Here's the drawing with two shaded views (mm, measured from the low corner). I have some questions. A direction names the side the tool comes from. Give positions to 0.01 mm unless a question says otherwise; leave off trailing zeros. Loops run counter-clockwise (first coordinate to the right, second up) from the corner with the lowest first, then second, coordinate; pieces in that order, holes last. Notation, with made-up numbers: (-39, 87) - (-32, 87) arc R23 cw to (-32, 111) - close; hole circle Ø9 at (2.25, 1). An arc over 180 degrees is marked (long way). Write each question's results on one line, items separated by ' | '. Start each with the question number.
1) If I drill on probe 1 along Y at (x, z) = (3, 1.9); probe 2 along Z at (x, y) = (3.1, 5.75); probe 3 along X at (y, z) = (3.35, 1.2), over which ranges is the centre line in solid material (lowest first)? Write a range as [from, to].
2) I'm going to push flat-ended pins straight in: pin 1 (3 mm diameter, centred on x = 3.5, y = 5, fed in from -Z); pin 2 (1 mm diameter, centred on y = 1, z = 2, fed in from +X); pin 3 (2 mm diameter, centred on y = 2, z = 4.5, fed in from +X). Where does each tip first touch, or does it pass through?
3) I want a section at A-A, the plane x = 3. Write out the boundary of the cut face in (y, z).
4) If we mould it in two halves opening along Y, with no side actions, what happens to the marked faces 1, 2 and 3? For each: +Y half, -Y half, draft (parallel to the pull), parting line (faces both ways), or undercut.
5) I want a section at C-C, the plane z = 4.35. Write out the boundary of the cut face in (x, y), and give its area (3 significant figures).
6) On a 3-axis mill with a long thin cutter (end or side, diameter ignored), from which of +Z, -Z, +X, -X, +Y, -Y can I reach the whole of each face in a straight line? I mean the marked faces 4 and 5. Say none if no direction works.
7) I want a section at D-D, the plane z = 1.2. Write out the boundary of the cut face in (x, y), and give its area (3 significant figures).
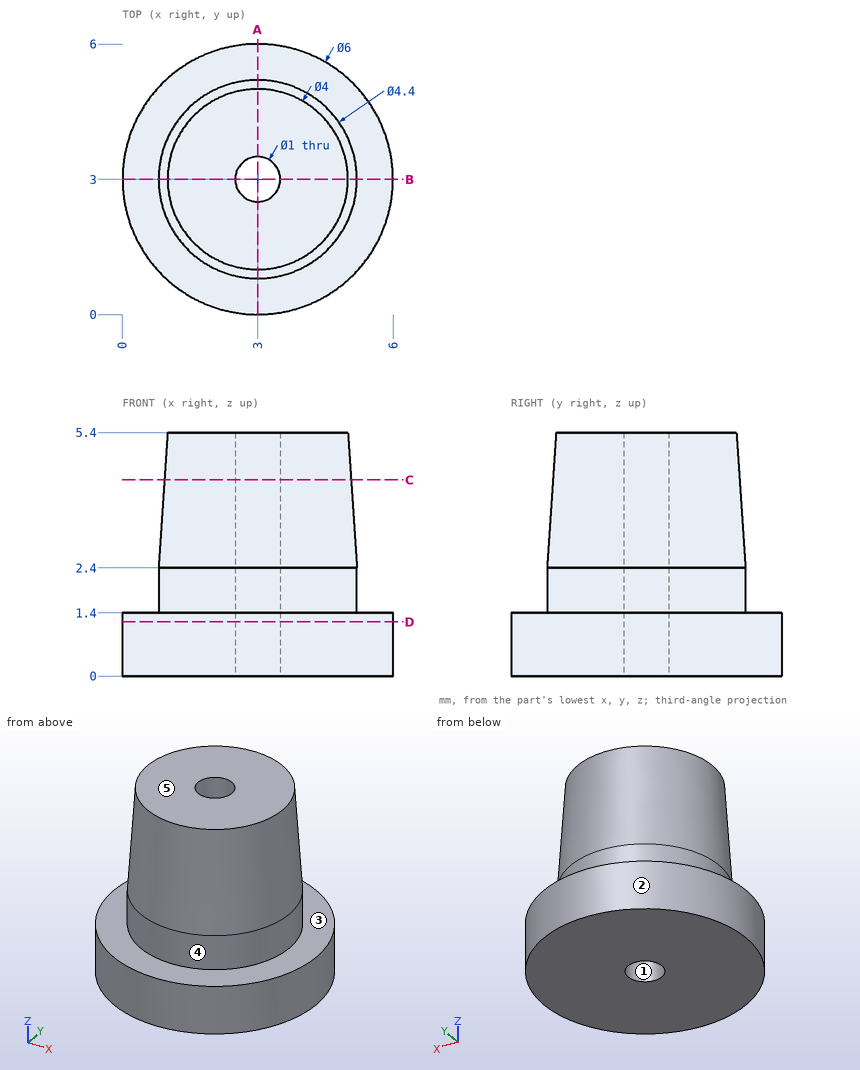
Answers:
1) probe 1: y = [0.8, 2.5], [3.5, 5.2] | probe 2: z = [0, 1.4] | probe 3: x = [0.02, 2.64], [3.36, 5.98]
2) pin 1: stops at z = 0 | pin 2: stops at x = 4.61 | pin 3: stops at x = 5.09
3) outline: (0, 0) - (2.5, 0) - (2.5, 5.4) - (1, 5.4) - (0.8, 2.4) - (0.8, 1.4) - (0, 1.4) - close; (3.5, 0) - (6, 0) - (6, 1.4) - (5.2, 1.4) - (5.2, 2.4) - (5, 5.4) - (3.5, 5.4) - close
4) face 1: undercut | face 2: parting line | face 3: draft
5) outline: circle Ø4.14 at (3, 3); hole circle Ø1 at (3, 3) | area: 12.7 mm2
6) face 4: +Z | face 5: +Z, +X, -X, +Y, -Y
7) outline: circle Ø6 at (3, 3); hole circle Ø1 at (3, 3) | area: 27.5 mm2
